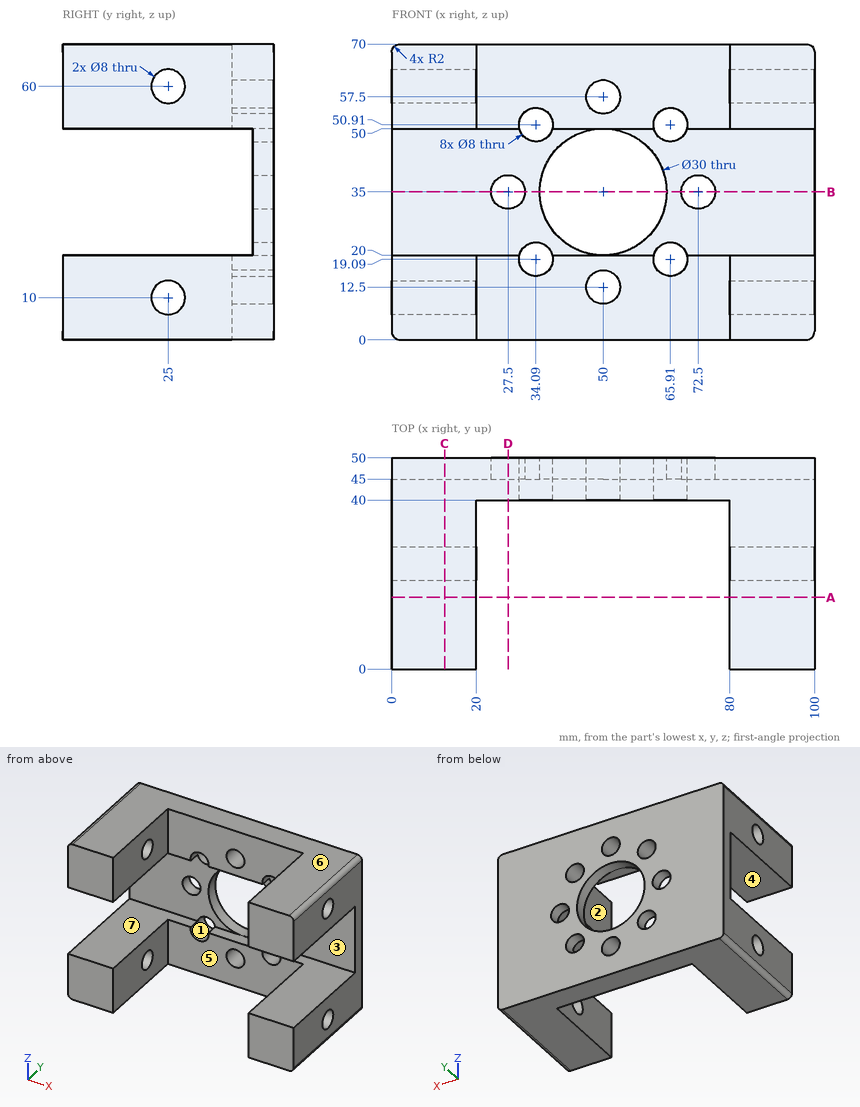
For this review, use the dimensioned drawing (mm, ordinates from the lowest corner) and the shaded views. A direction names the side the tool comes from. Round coordinates to 2 decimals unless told otherwise and drop trailing zeros. Order: outer loops, then holes, each group sorted by start corner. A loop starts at its lowest first (then second) coordinate and runs counter-clockwise, first axis right, second up. Notation, with made-up numbers: M 59,-36.5 L 97,-36.5 A14 ccw 97,-20.5 Z; hole C -34,34.5 d11. An arc over 180 degrees is marked long. Use a Markdown table: item, result. Add a question column.
Item 1: Add section C-C, the plane x = 12.5. Give the boundary of the cut face in (y, z).
Item 2: Insertion check: pin 1 (13 mm diameter, centred on x = 50, z = 12.5, fed in from -Y). The pin has a flat end and moves straight along its axis. Give the tip position at first contact, or say it passes through.
Item 3: Mouldability with a two-part tool opening along Z and no side actions: class the marked faces 4, 5, 6 and 7 as released by +Z, released by -Z, zero draft, split by the parting line, or undercut.
Item 4: Tool access review of the marked faces 1, 2 and 3: name each direction out of +Z, -Z, +X, -X, +Y, -Y from which nothing blocks a thin tool from reaching the whole face with its end or side.
Item 5: Add section D-D, the plane x = 27.5. Give the boundary of the cut face in (y, z).
Item 6: To check wall thickness, follow line 1 along X through (y, z) = (12.5, 4); line 2 along Z through (x, y) = (80.5, 31.5); line 3 along X through (y, z) = (42.25, 57.5). State the ranges of each line that lie inside material, in increasing order.
Item 7: Add section B-B, the plane z = 35. Give the boundary of the cut face in (x, y), then the cut area to 3 significant figures.
Item 8: Add section A-A, the plane y = 17. Give the boundary of the cut face in (x, z), then the cut area to 3 significant figures.
Geometry results:
| question | item | result |
|---|---|---|
| 1 | outline | M 0,0 L 50,0 L 50,70 L 0,70 L 0,50 L 45,50 L 45,20 L 0,20 Z; hole C 25,10 d8; hole C 25,60 d8 |
| 2 | pin 1 | stops at y = 40 |
| 3 | face 4 | undercut |
| 3 | face 5 | zero draft |
| 3 | face 6 | released by +Z |
| 3 | face 7 | undercut |
| 4 | face 1 | +Y, -Y |
| 4 | face 2 | +Z, -Z, -Y |
| 4 | face 3 | +X, -X, -Y |
| 5 | outline | M 40,0 L 50,0 L 50,31 L 45,31 L 45,20 L 40,20 Z; M 40,50 L 45,50 L 45,39 L 50,39 L 50,70 L 40,70 Z |
| 6 | line 1 | x = 0 to 20, 80 to 100 |
| 6 | line 2 | z = 0 to 20, 50 to 70 |
| 6 | line 3 | x = 0 to 46, 54 to 100 |
| 7 | outline | M 0,45 L 23.5,45 L 23.5,50 L 0,50 Z; M 31.5,45 L 35,45 L 35,50 L 31.5,50 Z; M 65,45 L 68.5,45 L 68.5,50 L 65,50 Z; M 76.5,45 L 100,45 L 100,50 L 76.5,50 Z |
| 7 | area | 270 mm² |
| 8 | outline | M 0,2 A2 ccw 2,0 L 20,0 L 20,20 L 0,20 Z; M 0,50 L 20,50 L 20,70 L 2,70 A2 ccw 0,68 Z; M 80,0 L 98,0 A2 ccw 100,2 L 100,20 L 80,20 Z; M 80,50 L 100,50 L 100,68 A2 ccw 98,70 L 80,70 Z |
| 8 | area | 1,600 mm² |
